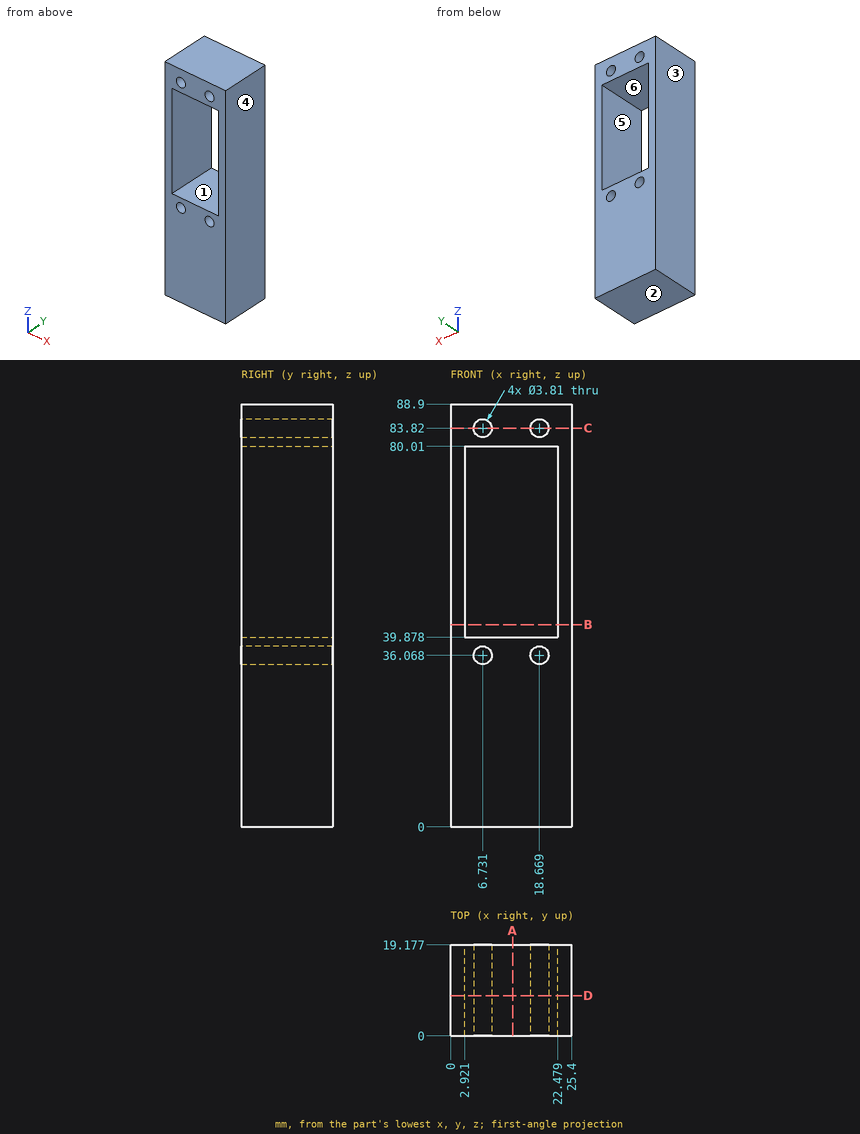
The drawing under review shows one solid part. Ordinate dimensions are in mm from its lowest x, y, z. A direction names the side the tool comes from. Give positions to 0.01 mm unless a question says otherwise; leave off trailing zeros. Write each loop counter-clockwise with the first axis right and the second up, starting at its lowest first coordinate (ties: lowest second). Pieces come first, ordered by that corner, then holes. Notation, with made-up numbers: (13, 26.5) -> (65, 26.5) arc R17 cw to (65, 55.5) -> close; hole circle Ø10 at (11, 16.25). An arc over 180 degrees is marked (long way). Answer in a Markdown table with one row per item.
(1) To check wall thickness, follow probe 1 along X at (y, z) = (6.25, 83.82); probe 2 along Z at (x, y) = (14, 1); probe 3 along X at (y, z) = (10, 73.5). State the ranges of each line that lie inside material, in increasing order.
Results:
| item | result |
|---|---|
| probe 1 | 0 to 4.83, 8.64 to 16.76, 20.57 to 25.4 |
| probe 2 | 0 to 39.88, 80.01 to 88.9 |
| probe 3 | 0 to 2.92, 22.48 to 25.4 |
(2) Mouldability with a two-part tool opening along X and no side actions: class the marked faces 3, 4, 5 and 6 as +X half, -X half, draft (parallel to the pull), parting line (faces both ways), or undercut.
Results:
| item | result |
|---|---|
| face 3 | -X half |
| face 4 | +X half |
| face 5 | undercut |
| face 6 | undercut |
(3) Clearance check with a flat-ended pin moving along its axis: pin 1 (3 mm diameter, centred on x = 18.669, z = 36.068, fed in from +Y). State where the tip first meets the part, or that it passes through.
Results:
| item | result |
|---|---|
| pin 1 | through |
(4) Consider section B-B (z = 42.5). State the section outline as (x, y) points, then the cut area to 3 significant figures.
Results:
| item | result |
|---|---|
| outline | (0, 0) -> (2.92, 0) -> (2.92, 19.18) -> (0, 19.18) -> close; (22.48, 0) -> (25.4, 0) -> (25.4, 19.18) -> (22.48, 19.18) -> close |
| area | 112 mm2 |
(5) Consider section D-D (y = 8.5). State the section outline as (x, z) points (3 decimals), then the cut area to 3 significant figures.
Results:
| item | result |
|---|---|
| outline | (0, 0) -> (25.4, 0) -> (25.4, 88.9) -> (0, 88.9) -> close; hole (2.921, 39.878) -> (22.479, 39.878) -> (22.479, 80.01) -> (2.921, 80.01) -> close; hole circle Ø3.81 at (6.731, 36.068); hole circle Ø3.81 at (6.731, 83.82); hole circle Ø3.81 at (18.669, 36.068); hole circle Ø3.81 at (18.669, 83.82) |
| area | 1,430 mm2 |
(6) Consider section A-A (x = 13). State the section outline as (y, z) points.
Results:
| item | result |
|---|---|
| outline | (0, 0) -> (19.18, 0) -> (19.18, 39.88) -> (0, 39.88) -> close; (0, 80.01) -> (19.18, 80.01) -> (19.18, 88.9) -> (0, 88.9) -> close |
(7) For the marked faces 1 and 2, list the 3-axis set-ups (+Z, -Z, +X, -X, +Y, -Y) from which the entire face can be reached by the end or side of a thin tool; tool diameter is ignored.
Results:
| item | result |
|---|---|
| face 1 | +Y, -Y |
| face 2 | -Z, +X, -X, +Y, -Y |
(8) Consider section C-C (z = 83.82). State the section outline as (x, y) points, then the cut area to 3 significant figures.
Results:
| item | result |
|---|---|
| outline | (0, 0) -> (4.83, 0) -> (4.83, 19.18) -> (0, 19.18) -> close; (8.64, 0) -> (16.76, 0) -> (16.76, 19.18) -> (8.64, 19.18) -> close; (20.57, 0) -> (25.4, 0) -> (25.4, 19.18) -> (20.57, 19.18) -> close |
| area | 341 mm2 |
